```python
from build123d import *

# Parameters (mm, degrees)
F0_W     = 40
F0_H     = 40
F1_DEPTH = 20
F3_DEPTH = 20


with BuildPart() as f1:
    # F0 (on Front) → F1 (new body)
    with BuildSketch(Plane.XZ):
        with Locations((20, 20)):
            Rectangle(F0_W, F0_H)
    extrude(amount=F1_DEPTH)

    # F2 (on face) → F3 (join)
    with BuildSketch(Plane.XZ.offset(20)):
        Polygon((20, 40), (0, 0), (40, 0), align=None)
    extrude(amount=F3_DEPTH)


solid = f1.part
```
Input: part model. Units: mm. Frame: model coordinates. A direction names the side the tool comes from. Round coordinates to 2 decimals unless told otherwise and drop trailing zeros. Order: outer loops, then holes, each group sorted by start corner. A loop starts at its lowest first (then second) coordinate and runs counter-clockwise, first axis right, second up. Notation, with made-up numbers: (77.25, -6) - (131.25, -6) arc R17 cw to (131.25, 10) - close; hole circle Ø8 at (-25.75, -36). An arc over 180 degrees is marked (long way). Answer in a Markdown table with one row per item.
Item 1: Line query: line 1 (Y direction, x = 9.5, z = 22); line 2 (Z direction, x = 14.5, y = -33.5); line 3 (Z direction, x = 18, y = -27). Output: solid intervals per line, ascending.
Model answer:
| item | result |
|---|---|
| line 1 | y = -20 to 0 |
| line 2 | z = 0 to 29 |
| line 3 | z = 0 to 36 |
Item 2: Section query A-A (z = 22). Return the cut outline in (x, y), then the cut area to 3 significant figures.
Model answer:
| item | result |
|---|---|
| outline | (0, -20) - (11, -20) - (11, -40) - (29, -40) - (29, -20) - (40, -20) - (40, 0) - (0, 0) - close |
| area | 1,160 mm² |
Item 3: Section query C-C (z = 28.5). Return the cut outline in (x, y), then the cut area to 3 significant figures.
Model answer:
| item | result |
|---|---|
| outline | (0, -20) - (14.25, -20) - (14.25, -40) - (25.75, -40) - (25.75, -20) - (40, -20) - (40, 0) - (0, 0) - close |
| area | 1,030 mm² |
Item 4: Pin query (flat end, axial travel): pin 1 (6 mm diameter, centred on x = 22.5, y = -27, fed in from -Z); pin 2 (2 mm diameter, centred on x = 36, y = -25.5, fed in from +Z). Return the tip coordinate at first contact, or that it passes through.
Model answer:
| item | result |
|---|---|
| pin 1 | stops at z = 0 |
| pin 2 | stops at z = 10 |
Item 5: Reachability of faces 1 (the flat face through (8, -20, 25)), 2 (the flat face through (34, -20, 29)), 3 (the flat face through (20, -10, 40)) from +Z, -Z, +X, -X, +Y, -Y: full face, straight path, thin tool, end or side. Return the list, or none.
Model answer:
| item | result |
|---|---|
| face 1 | +Z, -X, -Y |
| face 2 | +Z, +X, -Y |
| face 3 | +Z, +X, -X, +Y, -Y |
Item 6: Section query D-D (y = -28). Return the cut outline in (x, z).
Model answer:
| item | result |
|---|---|
| outline | (0, 0) - (40, 0) - (20, 40) - close |
Item 7: Section query B-B (x = 8). Return the cut outline in (y, z).
Model answer:
| item | result |
|---|---|
| outline | (-40, 0) - (0, 0) - (0, 40) - (-20, 40) - (-20, 16) - (-40, 16) - close |
